Read the model definition and answer for the solid it produces. Units are mm, in the model's axes. A direction names the side the tool comes from. Round coordinates to 2 decimals unless told otherwise and drop trailing zeros. Write each loop counter-clockwise with the first axis right and the second up, starting at its lowest first coordinate (ties: lowest second). Pieces come first, ordered by that corner, then holes. Notation, with made-up numbers: (-24, 0) - (16, 0) arc R21 ccw to (16, 13) - close; hole circle Ø1 at (38.5, 6.25). An arc over 180 degrees is marked (long way). One line per item, written item: value. Start each with the question number.
(1) For faces 1 (the face through (455.382, 72, 46)), 2 (the face through (368, 32, 0)), 3 (the face through (724, 60, 44)), determine the directions among +Z, -Z, +X, -X, +Y, -Y from which every point of the face is accessible in a straight line to the end or side of a thin tool.
(2) A cutting plane is placed at B-B, the plane x = -33.5. Determine the outline of the cut face in (y, z).
(3) A cutting plane is placed at A-A, the plane z = 36. Determine the outline of the cut face in (x, y).
(4) Find the intervals of material crossed by L1, parallel to X at y = 82, z = 67; L2, parallel to X at y = 82, z = 25; L3, parallel to Y at x = -43.5, z = 63, in increasing order.
(5) Flat-ended cylindrical pins translate along their axes: pin 1 Ø8 at (x, z) = (495.38, 23) entering from -Y; pin 2 Ø5.5 at (x, z) = (537.38, 67) entering from +Y; pin 3 Ø7.5 at (y, z) = (66.5, 40) entering from +X; pin 4 Ø12 at (x, z) = (399, 67) entering from +Y. Find the tip coordinate at first contact, or state that the pin passes through.
from build123d import *

# Parameters (mm, degrees)
SKETCH1_W           = 1000
SKETCH1_H           = 90
BOSS_EXTRUDE1_DEPTH = 60
SKETCH2_W           = 122
SKETCH2_H           = 90
BOSS_EXTRUDE2_DEPTH = 25
SKETCH3_R           = 3
CUT_EXTRUDE1_DEPTH  = 10


with BuildPart() as part:
    # Sketch1 → Boss-Extrude1 (new body)
    with BuildSketch(Plane(origin=(0, 0, 0), x_dir=(1, 0, 0), z_dir=(0, 1, 0))):
        with Locations((374.694533762, -45)):
            Rectangle(SKETCH1_W, SKETCH1_H)
    extrude(amount=BOSS_EXTRUDE1_DEPTH)

    # Sketch2 → Boss-Extrude2 (add)
    with BuildSketch(Plane(origin=(0, 60, 0), x_dir=(1, 0, 0), z_dir=(0, 1, 0))):
        with Locations((516.382198595, -45)):
            Rectangle(SKETCH2_W, SKETCH2_H)
    extrude(amount=BOSS_EXTRUDE2_DEPTH)

    # Sketch3 → Cut-Extrude1 (cut)
    with BuildSketch(Plane(origin=(0, 85, 0), x_dir=(1, 0, 0), z_dir=(0, 1, 0))):
        with Locations((495.382198595, -23)):
            Circle(SKETCH3_R)
        with Locations((537.382198595, -23)):
            Circle(SKETCH3_R)
        with Locations((537.382198595, -67)):
            Circle(SKETCH3_R)
        with Locations((495.382198595, -67)):
            Circle(SKETCH3_R)
    extrude(amount=-CUT_EXTRUDE1_DEPTH, mode=Mode.SUBTRACT)


solid = part.part
Here are the results:
1. face 1: +Z, -Z, -X, +Y
1. face 2: -Z, +X, -X, +Y, -Y
1. face 3: +Z, -Z, +X, +Y
2. outline: (0, 0) - (60, 0) - (60, 90) - (0, 90) - close
3. outline: (-125.31, 0) - (874.69, 0) - (874.69, 60) - (577.38, 60) - (577.38, 85) - (455.38, 85) - (455.38, 60) - (-125.31, 60) - close
4. L1: 455.38 to 492.38, 498.38 to 534.38, 540.38 to 577.38
4. L2: 455.38 to 493.15, 497.62 to 535.15, 539.62 to 577.38
4. L3: 0 to 60
5. pin 1: y = 0
5. pin 2: y = 75
5. pin 3: x = 577.38
5. pin 4: y = 60
